For this review, take the finished solid that the model builds, in its own axes (mm). A direction names the side the tool comes from. Give positions to 0.01 mm unless a question says otherwise; leave off trailing zeros. Answer as CSV lines item,"result". Start each with the question number.
1. Clearance check with flat-ended pins moving along their axes: P1, Ø3, axis at x = 46.5, y = 38, coming from the +Z side; P2, Ø4, axis at y = 38.5, z = -38.5, coming from the +X side; P3, Ø1.5, axis at x = 47, y = 7.5, coming from the +Z side. State where each tip first meets the part, or that it passes through.
2. Mouldability with a two-part tool opening along X and no side actions: class faces 6 (the cylindrical face through (51.622, 53.514, -47.707)), 7 (the cylindrical face through (66.77, 4.01, 15.37)), 8 (the flat face through (44.473, 28.473, -33.12)), 9 (the flat face through (34, 52.5, -10)) as pulls with the +X half, pulls with the -X half, needs draft (parallel to the pull), parting line crosses it, or undercut.
3. Machinability: for faces 1 (the flat face through (34, 57.5, -17)), 2 (the flat face through (26.4, 4, 1)), 3 (the cylindrical face through (1.352, 3.768, 4.292)), 4 (the cylindrical face through (50.775, 56.645, -2.497)), 5 (the cylindrical face through (43.26, 51.36, -33.19)), which of the approach directions +Z, -Z, +X, -X, +Y, -Y give a long, thin tool a straight path to every point of the face, cutting with its end or side? Answer none if there is none.
4. We need section B-B, the plane z = 0. State how many separate pieces and enclosed holes the cut face has, and give its area (3 significant figures).
5. For line 1 along Y through (x, z) = (51.5, -11); line 2 along X through (y, z) = (3, 0); line 3 along X through (y, z) = (54.4, 0), list the stretches that pass through material, from the lowest coordinate up.
from build123d import *

# Parameters (mm, degrees)
SALIENTE_EXTRUIR2_DEPTH = 5
CROQUIS2_R              = 4.5
CORTAR_EXTRUIR1_DEPTH   = 2.5
SALIENTE_EXTRUIR3_DEPTH = 47.5
SALIENTE_EXTRUIR4_DEPTH = 5
CROQUIS6_R              = 10.5
CORTAR_EXTRUIR2_DEPTH   = 2.5
CROQUIS7_W              = 26.576799325
CROQUIS7_H              = 47.5
CROQUIS7_W_2            = 20
CORTAR_EXTRUIR3_DEPTH   = 12.5
REDONDEO1_R             = 15
REDONDEO2_R             = 3
REDONDEO3_R             = 4


with BuildPart() as part:
    # Croquis1 → Saliente-Extruir2 (new body)
    with BuildSketch(Plane(origin=(0, 0, 0), x_dir=(1, 0, 0), z_dir=(0, 1, 0))):
        Polygon((-4.276899691, -21.499026234), (-21.499026234, 4.276899691), (40.72350463, 45.850742798), (52.672201475, 53.834237539), (91.499026234, -4.276899691), (65.723100309, -21.499026234), (44.118402092, 10.836185071), align=None)
    extrude(amount=SALIENTE_EXTRUIR2_DEPTH)

    # Croquis2 → Cortar-Extruir1 (cut)
    with BuildSketch(Plane(origin=(0, 5, 0), x_dir=(1, 0, 0), z_dir=(0, 1, 0))):
        with Locations(Location((0, 0, 0), (0, 0, 270))):
            Circle(CROQUIS2_R)
        with Locations(Location((70, 0, 0), (0, 0, 270))):
            Circle(CROQUIS2_R)
    extrude(amount=-CORTAR_EXTRUIR1_DEPTH, mode=Mode.SUBTRACT)

    # Croquis4 → Saliente-Extruir3 (add)
    with BuildSketch(Plane(origin=(0, 5, 0), x_dir=(1, 0, 0), z_dir=(0, 1, 0))):
        Polygon((52.672201475, 53.834237539), (47.968631923, 50.691558194), (39.41483254, 7.693505725), (44.118402092, 10.836185071), (47.261081438, 6.132615519), (55.814880821, 49.130667987), align=None)
    extrude(amount=SALIENTE_EXTRUIR3_DEPTH)

    # Croquis5 → Saliente-Extruir4 (add)
    with BuildSketch(Plane(origin=(0, 52.5, 0), x_dir=(1, 0, 0), z_dir=(0, 1, 0))):
        Polygon((-21.499026234, 4.276899691), (-4.276899691, -21.499026234), (44.118402092, 10.836185071), (65.723100309, -21.499026234), (91.499026234, -4.276899691), (52.672201475, 53.834237539), align=None)
    extrude(amount=SALIENTE_EXTRUIR4_DEPTH)

    # Croquis6 → Cortar-Extruir2 (cut)
    with BuildSketch(Plane.XZ.offset(-52.5)):
        with Locations(Location((0, 0, 0), (0, 0, 270))):
            Circle(CROQUIS6_R)
        with Locations(Location((70, 0, 0), (0, 0, 270))):
            Circle(CROQUIS6_R)
    extrude(amount=-CORTAR_EXTRUIR2_DEPTH, mode=Mode.SUBTRACT)

    # Croquis7 → Cortar-Extruir3 (cut)
    with BuildSketch(Plane(origin=(36.442132095, 0, 7.249600136), x_dir=(-0.19511127576179904, 0, 0.9807811122113861), z_dir=(-0.9807811122113861, 0, -0.19511127576179904))):
        with Locations((-64.364943459, 28.75)):
            Rectangle(CROQUIS7_W, CROQUIS7_H)
        with Locations((-21.076543796, 28.75)):
            Rectangle(CROQUIS7_W_2, CROQUIS7_H)
    extrude(amount=-CORTAR_EXTRUIR3_DEPTH, mode=Mode.SUBTRACT)

    # Redondeo1
    redondeo1_edges = [part.edges().sort_by_distance(p)[0] for p in [
        (-4.276899691, 2.5, 21.499026234),
        (-21.499026234, 2.5, -4.276899691),
        (52.672201475, 55, -53.834237539),
        (91.499026234, 2.5, 4.276899691),
        (65.723100309, 2.5, 21.499026234),
        (-21.499026234, 55, -4.276899691),
        (-4.276899691, 55, 21.499026234),
        (65.723100309, 55, 21.499026234),
        (91.499026234, 55, 4.276899691),
        (52.672201475, 2.5, -53.834237539),
    ]]
    fillet(redondeo1_edges, radius=REDONDEO1_R)

    # Redondeo2
    redondeo2_edges = [part.edges().sort_by_distance(p)[0] for p in [
        (50.754107682, 0, -0.904690529),
        (15.58658762, 0, -29.055568615),
        (26.156862311, 0, 1.164777064),
        (-12.887962963, 0, 8.611063271),
        (72.085613855, 0, -24.778668924),
        (78.611063271, 0, 12.887962963),
        (85.405233658, 0, 3.064633643),
        (66.935366357, 0, 15.405233658),
        (-3.064633643, 0, 15.405233658),
        (-15.405233658, 0, -3.064633643),
        (51.459935426, 0, -47.740444963),
        (15.58658762, 57.5, -29.055568615),
        (72.085613855, 57.5, -24.778668924),
        (-12.887962963, 57.5, 8.611063271),
        (26.156862311, 57.5, 1.164777064),
        (78.611063271, 57.5, 12.887962963),
        (-15.405233658, 57.5, -3.064633643),
        (-3.064633643, 57.5, 15.405233658),
        (66.935366357, 57.5, 15.405233658),
        (85.405233658, 57.5, 3.064633643),
        (51.459935426, 57.5, -47.740444963),
        (50.754107682, 57.5, -0.904690529),
    ]]
    fillet(redondeo2_edges, radius=REDONDEO2_R)

    # Redondeo3
    redondeo3_edges = [part.edges().sort_by_distance(p)[0] for p in [
        (46.42864065, 52.5, -22.449241949),
        (42.505516202, 28.75, -23.229687052),
        (50.351765099, 28.75, -21.668796846),
        (46.42864065, 5, -22.449241949),
        (52.302877857, 52.5, -31.476607968),
        (44.456628959, 52.5, -33.037498174),
        (52.302877857, 5, -31.476607968),
        (44.456628959, 5, -33.037498174),
        (50.330866166, 5, -42.064864193),
        (46.407741717, 28.75, -42.845309296),
        (54.253990614, 28.75, -41.28441909),
        (50.330866166, 52.5, -42.064864193),
    ]]
    fillet(redondeo3_edges, radius=REDONDEO3_R - 0.0001)  # a hair under: the kernel refuses the full size


solid = part.part
Result set:
1,P1,"z = -22.37"
1,P2,"x = 53.55"
1,P3,"z = -21.68"
2,face 6,"parting line crosses it"
2,face 7,"undercut"
2,face 8,"pulls with the -X half"
2,face 9,"needs draft"
3,face 1,"+Z, -Z, +X, -X, +Y"
3,face 2,"+Z, +Y, -Y"
3,face 3,"none"
3,face 4,"+Z, +Y"
3,face 5,"-Z, -X"
4,separate pieces,"4"
4,enclosed holes,"0"
4,area,"610 mm2"
5,line 1,"0 to 5, 52.5 to 57.5"
5,line 2,"-15.69 to -4.5, 4.5 to 27.9, 51.36 to 65.5, 74.5 to 85.69"
5,line 3,"-15.69 to -10.5, 10.5 to 27.9, 51.36 to 59.5, 80.5 to 85.69"
